Check sheet for the drawn part. Datum: minimum x, y, z corner. Units: mm. A direction names the side the tool comes from. Round coordinates to 2 decimals unless told otherwise and drop trailing zeros. Order: outer loops, then holes, each group sorted by start corner. A loop starts at its lowest first (then second) coordinate and runs counter-clockwise, first axis right, second up. Notation, with made-up numbers: (18, 44) - (67, 44) arc R19 cw to (67, 67) - close; hole circle Ø11 at (71.25, 44). An arc over 180 degrees is marked (long way). Write each question's results on one line, items separated by ' | '.
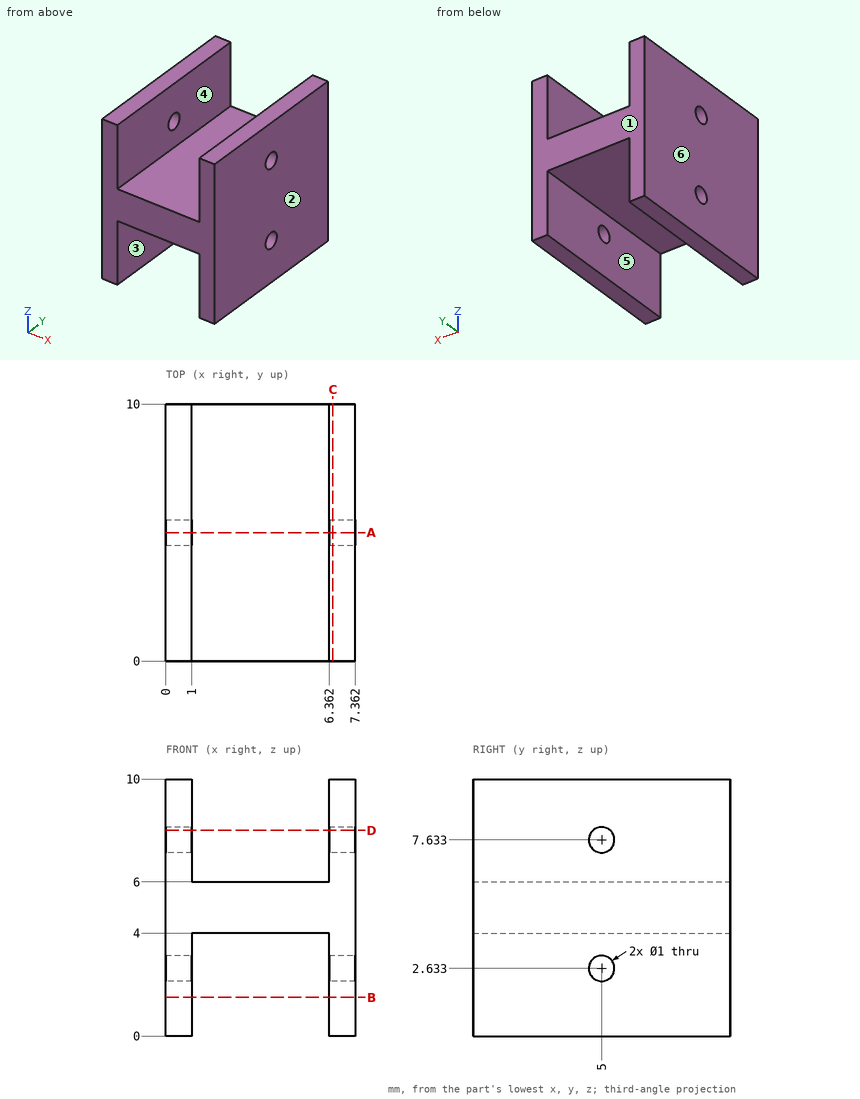
(1) Section check D-D (z = 8). Record the cut outline in (x, y).
Answers follow:
outline: (0, 0) - (1, 0) - (1, 4.66) - (0, 4.66) - close; (0, 5.34) - (1, 5.34) - (1, 10) - (0, 10) - close; (6.36, 0) - (7.36, 0) - (7.36, 4.66) - (6.36, 4.66) - close; (6.36, 5.34) - (7.36, 5.34) - (7.36, 10) - (6.36, 10) - close
(2) Section check B-B (z = 1.5). Record the cut outline in (x, y).
Answers follow:
outline: (0, 0) - (1, 0) - (1, 10) - (0, 10) - close; (6.36, 0) - (7.36, 0) - (7.36, 10) - (6.36, 10) - close
(3) Section check A-A (y = 5). Record the cut outline in (x, z).
Answers follow:
outline: (0, 0) - (1, 0) - (1, 2.13) - (0, 2.13) - close; (0, 3.13) - (1, 3.13) - (1, 4) - (6.36, 4) - (6.36, 3.13) - (7.36, 3.13) - (7.36, 7.13) - (6.36, 7.13) - (6.36, 6) - (1, 6) - (1, 7.13) - (0, 7.13) - close; (0, 8.13) - (1, 8.13) - (1, 10) - (0, 10) - close; (6.36, 0) - (7.36, 0) - (7.36, 2.13) - (6.36, 2.13) - close; (6.36, 8.13) - (7.36, 8.13) - (7.36, 10) - (6.36, 10) - close
(4) Depth check by flat-ended pin: pin 1 Ø1.6 at (x, y) = (3.5, 6.5) entering from +Z. Enter the tip coordinate at first touch or a pass-through.
Answers follow:
pin 1: z = 6
(5) Access from +Z, -Z, +X, -X, +Y, -Y to the whole of each face (thin tool, end or side, straight path). Record for the marked faces 4, 5 and 6.
Answers follow:
face 4: +Z, +Y, -Y | face 5: -Z, +Y, -Y | face 6: +Z, -Z, -X, +Y, -Y
(6) Draft check along X on the marked faces 1, 2 and 3. Enter one of: released by +X, released by -X, zero draft, split by the parting line, or undercut.
Answers follow:
face 1: zero draft | face 2: released by +X | face 3: undercut
(7) Material ranges on line 1 (X direction, y = 9.25, z = 6.25); line 2 (Z direction, x = 6.25, y = 0.75), recorded low to high.
Answers follow:
line 1: 0 to 1, 6.36 to 7.36 | line 2: 4 to 6
(8) Section check C-C (x = 6.5). Record the cut outline in (y, z).
Answers follow:
outline: (0, 0) - (10, 0) - (10, 10) - (0, 10) - close; hole circle Ø1 at (5, 2.63); hole circle Ø1 at (5, 7.63)
